Here's how the part is built. I have some questions about the finished solid (model axes, mm). A direction names the side the tool comes from. Round coordinates to 2 decimals unless told otherwise and drop trailing zeros. Order: outer loops, then holes, each group sorted by start corner. A loop starts at its lowest first (then second) coordinate and runs counter-clockwise, first axis right, second up. Notation, with made-up numbers: M 30,38.25 L 84,38.25 A24 cw 84,68.25 Z; hole C 0,33.5 d9. An arc over 180 degrees is marked long. Write item = value, one per line. Start each with the question number.
Item 1: I want a section at C-C, the plane y = 1.5. List the corners of the cut face in (x, z) for me, plus the area to 3 significant figures.
Item 2: For faces 4 (the face through (-3, 14, -1)), 5 (the face through (-9.182, -3.042, 21.894)), which set-ups out of +Z, -Z, +X, -X, +Y, -Y let a thin tool reach every point of the face, with its end or its side?
Item 3: I want a section at A-A, the plane z = 0. List the corners of the cut face in (x, y) for me, plus the area to 3 significant figures.
Item 4: Please list where these lines run through material, in increasing order: L1, parallel to X at y = 6, z = 0; L2, parallel to X at y = -3, z = -20.5; L3, parallel to Z at x = 23, y = -0.25.
Item 5: We'd pull the mould along X, two halves only. Please class faces 1 (the face through (25.107, -5.507, 13.059)), 2 (the face through (0, -6, 6)), 3 (the face through (-1.162, -3, -15)): pulls with the +X half, pulls with the -X half, needs draft (parallel to the pull), parting line crosses it, or undercut.
Item 6: I'm going to push flat-ended pins straight in: P1, Ø3, axis at x = -16.5, y = -2, coming from the +Z side; P2, Ø8, axis at x = 12, z = -1, coming from the +Y side; P3, Ø1.8, axis at y = -3.5, z = 11.5, coming from the +X side. Where does each tip first touch, or does it pass through?
Item 7: I want a section at B-B, the plane x = 0. State how many separate pieces and enclosed holes the cut face has, plus the area to 3 significant figures.
```python
from build123d import *

# Parameters (mm, degrees)
ENL_V_START             = -5.600001354
ENL_V_MAT_EXTRU_1_DEPTH = 11.200001454
ENL_V_MAT_EXTRU_3_DEPTH = 6


# Read off the part's stored shape, not the designer's step: Enlèv. mat.-Extru.1
with BuildPart() as part:
    # Esquisse1 → Révolution1 (revolve)
    with BuildSketch(Plane(origin=(0, 0, 0), x_dir=(0, 0, -1), z_dir=(1, 0, 0)), mode=Mode.PRIVATE) as r_volution1_sk:
        with BuildLine():
            Line((5.6, 0), (28.3, 0))
            Line((28.3, 0), (28.3, -1))
            ThreePointArc((28.3, -1), (26.3, -3), (28.3, -5))
            Line((28.3, -5), (28.3, -6))
            Line((28.3, -6), (2.6, -6))
            Line((2.6, -6), (2.6, 0))
            Line((2.6, 0), (2.6, 14))
            Line((2.6, 14), (5.6, 14))
            Line((5.6, 14), (5.6, 0))
        make_face()
    revolve(r_volution1_sk.sketch.rotate(Axis((0, 0, 0), (0, -1, 0)), 180), axis=Axis((0, 0, 0), (0, -1, 0)))

    # Enlèv. mat.-Extru.1 outline → Enlèv. mat.-Extru.1 (cut)
    with BuildSketch(Plane.XY.offset(ENL_V_START)):
        with BuildLine():
            add(Edge.make_bspline(
                [(0, 4.75), (0.6013076, 4.75), (1.181365788, 4.999070592), (2.001835342, 5.820169976), (2.249317955, 6.403361701), (2.250679092, 7.591483004), (2.003145141, 8.178489261), (1.180171672, 9.002154395), (0.594632574, 9.249370285), (-0.589857498, 9.250627181), (-1.17573609, 9.006205165), (-2.00609398, 8.175925788), (-2.249601609, 7.594858131), (-2.250397379, 6.408159453), (-2.004861685, 5.823479927), (-1.179421259, 4.996843653), (-0.6013076, 4.75), (0, 4.75)],
                knots=[0, 0, 0, 0, 0.125, 0.125, 0.25, 0.25, 0.375, 0.375, 0.5, 0.5, 0.625, 0.625, 0.75, 0.75, 0.875, 0.875, 1, 1, 1, 1], degree=3))
        make_face()
    extrude(amount=ENL_V_MAT_EXTRU_1_DEPTH, mode=Mode.SUBTRACT)

    # Esquisse3 → Enlèv. mat.-Extru.3 (cut)
    with BuildSketch(Plane.XZ.offset(6)):
        with BuildLine():
            Line((-1.161815326, -5.478155269), (-1.161815326, -24.455749626))
            ThreePointArc((-1.161815326, -24.455749626), (-1.383721907, -24.871278266), (-1.852471528, -24.917972746))
            Line((-1.852471528, -24.917972746), (-16.327607753, -18.947318365))
            ThreePointArc((-16.327607753, -18.947318365), (-16.6272717, -18.583004137), (-16.490504941, -18.131541855))
            Line((-16.490504941, -18.131541855), (-3.053336143, -4.694373057))
            ThreePointArc((-3.053336143, -4.694373057), (-2.143701032, -5.173446229), (-1.161815326, -5.478155269))
        make_face()
        with BuildLine():
            Line((-24.481484068, -1.16038833), (-5.478457714, -1.16038833))
            ThreePointArc((-5.478457714, -1.16038833), (-5.174004447, -2.142353374), (-4.695168234, -3.052113244))
            Line((-4.695168234, -3.052113244), (-18.114353895, -16.471298904))
            ThreePointArc((-18.114353895, -16.471298904), (-18.565088662, -16.608210375), (-18.929562681, -16.309772323))
            Line((-18.929562681, -16.309772323), (-24.943139464, -1.852415139))
            ThreePointArc((-24.943139464, -1.852415139), (-24.897424812, -1.382911668), (-24.481484068, -1.16038833))
        make_face()
        with BuildLine():
            Line((-18.131541855, 16.490504941), (-4.694373057, 3.053336143))
            ThreePointArc((-4.694373057, 3.053336143), (-5.173446229, 2.143701032), (-5.478155269, 1.161815326))
            Line((-5.478155269, 1.161815326), (-24.455749626, 1.161815326))
            ThreePointArc((-24.455749626, 1.161815326), (-24.871278266, 1.383721907), (-24.917972746, 1.852471528))
            Line((-24.917972746, 1.852471528), (-18.947318365, 16.327607753))
            ThreePointArc((-18.947318365, 16.327607753), (-18.583004137, 16.6272717), (-18.131541855, 16.490504941))
        make_face()
        with BuildLine():
            Line((-1.16038833, 24.481484068), (-1.16038833, 5.478457714))
            ThreePointArc((-1.16038833, 5.478457714), (-2.142353374, 5.174004447), (-3.052113244, 4.695168234))
            Line((-3.052113244, 4.695168234), (-16.471298904, 18.114353895))
            ThreePointArc((-16.471298904, 18.114353895), (-16.608210375, 18.565088662), (-16.309772323, 18.929562681))
            Line((-16.309772323, 18.929562681), (-1.852415139, 24.943139464))
            ThreePointArc((-1.852415139, 24.943139464), (-1.382911668, 24.897424812), (-1.16038833, 24.481484068))
        make_face()
        with BuildLine():
            Line((16.490504941, 18.131541855), (3.053336143, 4.694373057))
            ThreePointArc((3.053336143, 4.694373057), (2.143701032, 5.173446229), (1.161815326, 5.478155269))
            Line((1.161815326, 5.478155269), (1.161815326, 24.455749626))
            ThreePointArc((1.161815326, 24.455749626), (1.383721907, 24.871278266), (1.852471528, 24.917972746))
            Line((1.852471528, 24.917972746), (16.327607753, 18.947318365))
            ThreePointArc((16.327607753, 18.947318365), (16.6272717, 18.583004137), (16.490504941, 18.131541855))
        make_face()
        with BuildLine():
            Line((24.481484068, 1.16038833), (5.478457714, 1.16038833))
            ThreePointArc((5.478457714, 1.16038833), (5.174004447, 2.142353374), (4.695168234, 3.052113244))
            Line((4.695168234, 3.052113244), (18.114353895, 16.471298904))
            ThreePointArc((18.114353895, 16.471298904), (18.565088662, 16.608210375), (18.929562681, 16.309772323))
            Line((18.929562681, 16.309772323), (24.943139464, 1.852415139))
            ThreePointArc((24.943139464, 1.852415139), (24.897424812, 1.382911668), (24.481484068, 1.16038833))
        make_face()
        with BuildLine():
            Line((18.131541855, -16.490504941), (4.694373057, -3.053336143))
            ThreePointArc((4.694373057, -3.053336143), (5.173446229, -2.143701032), (5.478155269, -1.161815326))
            Line((5.478155269, -1.161815326), (24.455749626, -1.161815326))
            ThreePointArc((24.455749626, -1.161815326), (24.871278266, -1.383721907), (24.917972746, -1.852471528))
            Line((24.917972746, -1.852471528), (18.947318365, -16.327607753))
            ThreePointArc((18.947318365, -16.327607753), (18.583004137, -16.6272717), (18.131541855, -16.490504941))
        make_face()
        with BuildLine():
            Line((1.16038833, -24.481484068), (1.16038833, -5.478457714))
            ThreePointArc((1.16038833, -5.478457714), (2.142353374, -5.174004447), (3.052113244, -4.695168234))
            Line((3.052113244, -4.695168234), (16.471298904, -18.114353895))
            ThreePointArc((16.471298904, -18.114353895), (16.608210375, -18.565088662), (16.309772323, -18.929562681))
            Line((16.309772323, -18.929562681), (1.852415139, -24.943139464))
            ThreePointArc((1.852415139, -24.943139464), (1.382911668, -24.897424812), (1.16038833, -24.481484068))
        make_face()
    extrude(amount=-ENL_V_MAT_EXTRU_3_DEPTH, mode=Mode.SUBTRACT)


solid = part.part
```
Filled in:
q1.outline = C 0,0 d11.2; hole C 0,0 d5.2
q1.area = 77.3 mm^2
q2.face_4 = +Z, -Z, +X, -X, +Y
q2.face_5 = +Y, -Y
q3.outline = M -28.3,-6 L -2.6,-6 L -2.6,14 L -5.6,14 L -5.6,0 L -28.3,0 L -28.3,-1 A2 cw -28.3,-5 Z; M 2.6,-6 L 28.3,-6 L 28.3,-5 A2 cw 28.3,-1 L 28.3,0 L 5.6,0 L 5.6,14 L 2.6,14 Z
q3.area = 380 mm^2
q4.L1 = -5.6 to -2.6, 2.6 to 5.6
q4.L2 = -16.48 to -12.56, -1.16 to 1.16, 12.53 to 16.48
q4.L3 = -16.49 to -6.5, -1.16 to 1.16, 6.52 to 16.49
q5.face_1 = parting line crosses it
q5.face_2 = needs draft
q5.face_3 = undercut
q6.P1 = 23.75
q6.P2 = 0
q6.P3 = 24.38
q7.separate_pieces = 4
q7.enclosed_holes = 0
q7.area = 353 mm^2
